Can you work these out from the model? Positions are in its coordinate system, mm. Round coordinates to 2 decimals unless told otherwise and drop trailing zeros. Loops run counter-clockwise (first coordinate to the right, second up) from the corner with the lowest first, then second, coordinate; pieces in that order, holes last. Notation, with made-up numbers: M 86.25,-7 L 130.25,-7 A22 cw 130.25,20 Z; hole C 27,5 d3. An arc over 180 degrees is marked long. Return JSON: item names as keys, results as strings.
```python
from build123d import *

# Parameters (mm, degrees)
SKETCH_1_W      = 10
SKETCH_1_H      = 20
SKETCH_1_R      = 1.5
EXTRUDE_1_DEPTH = 2
FILLET_1_R      = 1


with BuildPart() as part:
    # 草图1 → 凸台-拉伸1 (new body)
    with BuildSketch(Plane.XY):
        with Locations((1.642083631, -11.90903272)):
            Rectangle(SKETCH_1_W, SKETCH_1_H)
        with Locations((1.642083631, -6.90903272)):
            Circle(SKETCH_1_R, mode=Mode.SUBTRACT)
        with Locations((1.642083631, -16.90903272)):
            Circle(SKETCH_1_R, mode=Mode.SUBTRACT)
    extrude(amount=EXTRUDE_1_DEPTH)

    # 圆角1
    fillet_1_edges = [part.edges().sort_by_distance(p)[0] for p in [
        (-3.357916369, -1.90903272, 1),
        (6.642083631, -1.90903272, 1),
        (6.642083631, -21.90903272, 1),
        (-3.357916369, -21.90903272, 1),
    ]]
    fillet(fillet_1_edges, radius=FILLET_1_R)


solid = part.part
```
Q1. Suppose I cut it at B-B, the plane z = 1.45. Please give me the cut outline in (x, y), plus the area to 3 significant figures.
Results:
{"outline": "M -3.36,-20.91 A1 ccw -2.36,-21.91 L 5.64,-21.91 A1 ccw 6.64,-20.91 L 6.64,-2.91 A1 ccw 5.64,-1.91 L -2.36,-1.91 A1 ccw -3.36,-2.91 Z; hole C 1.64,-16.91 d3; hole C 1.64,-6.91 d3", "area": "185 mm2"}
Q2. Thinking about a two-plate mould opening in X: for faces 1 (the cylindrical face through (2.448, -15.644, 0.986)), 2 (the flat face through (2, -12, 0)), 3 (the cylindrical face through (-3.07, -21.61, 1.01)), which applies, pulls with the +X half, pulls with the -X half, needs draft (parallel to the pull), parting line crosses it, or undercut?
Results:
{"face 1": "undercut", "face 2": "needs draft", "face 3": "pulls with the -X half"}
Q3. Suppose I cut it at D-D, the plane y = -16.25. Please give me the cut outline in (x, z).
Results:
{"outline": "M -3.36,0 L 0.29,0 L 0.29,2 L -3.36,2 Z; M 2.99,0 L 6.64,0 L 6.64,2 L 2.99,2 Z"}
Q4. Suppose I cut it at C-C, the plane x = 2.75. Please give me the cut outline in (y, z), plus the area to 3 significant figures.
Results:
{"outline": "M -21.91,0 L -17.92,0 L -17.92,2 L -21.91,2 Z; M -15.9,0 L -7.92,0 L -7.92,2 L -15.9,2 Z; M -5.9,0 L -1.91,0 L -1.91,2 L -5.9,2 Z", "area": "31.9 mm2"}
Q5. If I drill on line 1 along Y through (x, z) = (0.75, 1.25); line 2 along X through (y, z) = (-6.75, 1.1); line 3 along X through (y, z) = (-5.75, 1.3), over which ranges is the centre line in solid material (lowest first)?
Results:
{"line 1": "y = -21.91 to -18.11, -15.7 to -8.11, -5.7 to -1.91", "line 2": "x = -3.36 to 0.15, 3.13 to 6.64", "line 3": "x = -3.36 to 0.69, 2.59 to 6.64"}
Q6. Suppose I cut it at A-A, the plane y = -8. Please give me the cut outline in (x, z), plus the area to 3 significant figures.
Results:
{"outline": "M -3.36,0 L 0.61,0 L 0.61,2 L -3.36,2 Z; M 2.67,0 L 6.64,0 L 6.64,2 L 2.67,2 Z", "area": "15.9 mm2"}
